Source: three-view drawing plus pictorial views. Frame: mm from the lowest corner of the part. Give positions to 0.01 mm unless a question says otherwise; leave off trailing zeros. Write each loop counter-clockwise with the first axis right and the second up, starting at its lowest first coordinate (ties: lowest second). Pieces come first, ordered by that corner, then holes. Notation, with made-up numbers: (80, 65.25) -> (110, 65.25) arc R15 ccw to (110, 74.25) -> close; hole circle Ø4 at (48, 70). An arc over 180 degrees is marked (long way). Write item = value, one per line.
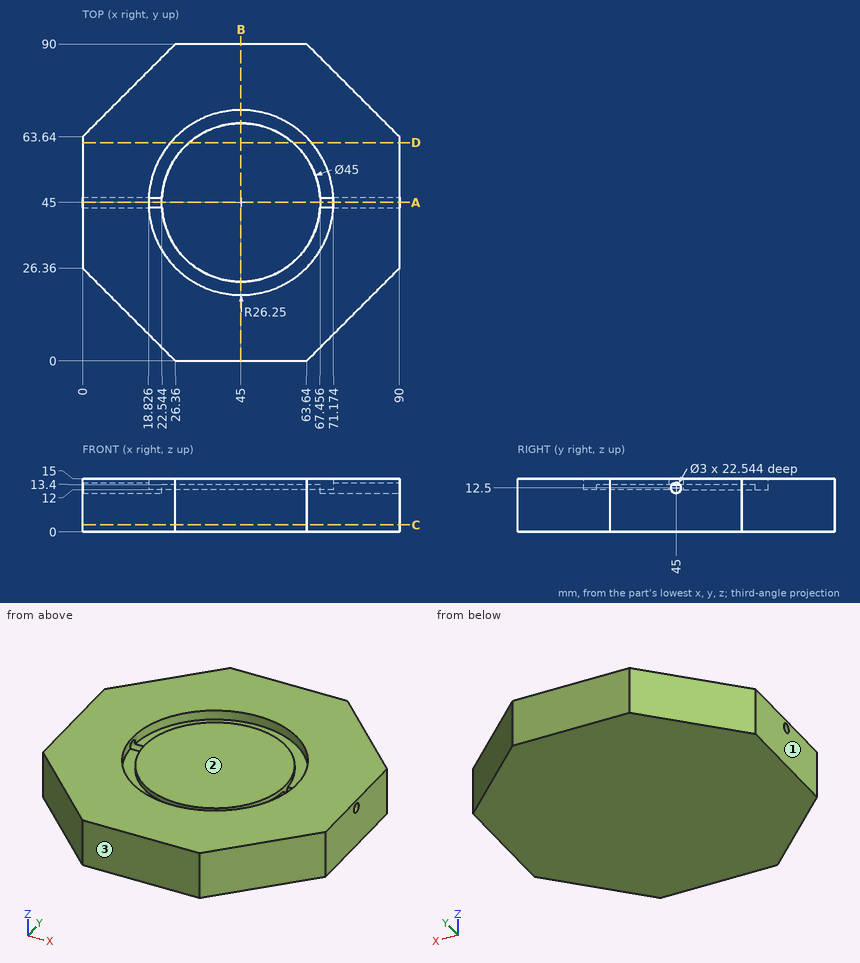
1) Cut plane C-C (z = 2). Return the cut outline in (x, y), then the cut area to 3 significant figures.
Computed:
outline = (0, 26.36) -> (26.36, 0) -> (63.64, 0) -> (90, 26.36) -> (90, 63.64) -> (63.64, 90) -> (26.36, 90) -> (0, 63.64) -> close
area = 6,710 mm²
2) Draft query along X for the marked faces 1, 2 and 3. Return one class per face: pulls with the +X half, pulls with the -X half, needs draft (parallel to the pull), parting line crosses it, or undercut.
Computed:
face_1 = pulls with the -X half
face_2 = undercut
face_3 = needs draft
3) Cut plane D-D (y = 62). Return the cut outline in (x, z).
Computed:
outline = (0, 0) -> (90, 0) -> (90, 15) -> (65, 15) -> (65, 12) -> (59.74, 12) -> (59.74, 13.4) -> (30.26, 13.4) -> (30.26, 12) -> (25, 12) -> (25, 15) -> (0, 15) -> close
4) Contact query for flat-ended pins moving along their axis: pin 1 (1 mm diameter, centred on y = 77, z = 9.5, fed in from +X); pin 2 (20 mm diameter, centred on x = 37, y = 56, fed in from +Z); pin 3 (5 mm diameter, centred on x = 41.5, y = 81, fed in from -Z); pin 4 (5 mm diameter, centred on x = 81, z = 2, fed in from -Y). Output: stop coordinate, or through.
Computed:
pin_1 = 77.14
pin_2 = 13.4
pin_3 = 0
pin_4 = 14.86
5) Cut plane A-A (y = 45). Return the cut outline in (x, z), then the cut area to 3 significant figures.
Computed:
outline = (0, 0) -> (90, 0) -> (90, 11) -> (67.5, 11) -> (67.5, 13.4) -> (22.5, 13.4) -> (22.5, 11) -> (0, 11) -> close; (0, 14) -> (18.83, 14) -> (18.83, 15) -> (0, 15) -> close; (71.17, 14) -> (90, 14) -> (90, 15) -> (71.17, 15) -> close
area = 1,140 mm²
6) Cut plane B-B (x = 45). Return the cut outline in (y, z).
Computed:
outline = (0, 0) -> (90, 0) -> (90, 15) -> (71.25, 15) -> (71.25, 12) -> (67.5, 12) -> (67.5, 13.4) -> (22.5, 13.4) -> (22.5, 12) -> (18.75, 12) -> (18.75, 15) -> (0, 15) -> close
7) Material intervals for L1, parallel to Z at x = 79, y = 45; L2, parallel to X at y = 38.5, z = 12.75; L3, parallel to Z at x = 33, y = 62.5, sorted ascending.
Computed:
L1 = 0 to 11, 14 to 15
L2 = 0 to 19.57, 23.46 to 66.54, 70.43 to 90
L3 = 0 to 13.4
